```python
from build123d import *

# Parameters (mm, degrees)
F3_R     = 1.75
F4_DEPTH = 12.5
F6_R     = 2
F8_DEPTH = 10
F2_W     = 25.478227
F2_H     = 5.5
F9_DEPTH = 1.3
F10_R    = 1


with BuildPart() as f1:
    # F0 (on Front) → F1 (revolve)
    with BuildSketch(Plane.XZ):
        Polygon((-9, -6), (0, -6), (0, 3), (-5, 3), (-5, -2), (-9, -2), align=None)
    revolve(axis=Axis((0, 0, -1.5), (0, 0, 1)))


with BuildPart() as f4:
    # F3 (on Top) → F4 (new body, symmetric)
    with BuildSketch(Plane.XY):
        Circle(F3_R)
    extrude(amount=F4_DEPTH, both=True)


with BuildPart() as f1_1:
    add(f1.part)

    # F5: cut F4
    add(f4.part, mode=Mode.SUBTRACT)

    # F6
    f6_edges = [f1_1.edges().sort_by_distance(p)[0] for p in [
        (5, 0, -2),
    ]]
    fillet(f6_edges, radius=F6_R)

    # F7 (on Top) → F8 (cut)
    with BuildSketch(Plane.XY):
        with BuildLine():
            ThreePointArc((-7.782135, -0.892736), (-7.266714, 0), (-7.782135, 0.892736))
            Line((-7.782135, 0.892736), (-10.312837, 2.353838))
            Line((-10.312837, 2.353838), (-10.499112, 2.339878))
            Line((-10.499112, 2.339878), (-10.499112, -2.339878))
            Line((-10.499112, -2.339878), (-10.312837, -2.353838))
            Line((-10.312837, -2.353838), (-7.782135, -0.892736))
        make_face()
        with BuildLine():
            Line((-10.474608, 2.447236), (-10.312837, 2.353838))
            Line((-10.312837, 2.353838), (-7.398805, 2.572214))
            ThreePointArc((-7.398805, 2.572214), (-6.547083, 3.152909), (-6.624118, 4.180869))
            Line((-6.624118, 4.180869), (-8.270253, 6.595307))
            Line((-8.270253, 6.595307), (-8.444138, 6.663552))
            Line((-8.444138, 6.663552), (-10.474608, 2.447236))
        make_face()
        Polygon((-10.499112, 2.396354), (-10.474608, 2.447236), (-10.499112, 2.461384), align=None)
        Polygon((-10.527328, 2.337764), (-10.499112, 2.339878), (-10.499112, 2.396354), align=None)
        with BuildLine():
            Line((-7.398805, -2.572214), (-10.312837, -2.353838))
            Line((-10.312837, -2.353838), (-10.474608, -2.447236))
            Line((-10.474608, -2.447236), (-8.444138, -6.663552))
            Line((-8.444138, -6.663552), (-8.270253, -6.595307))
            Line((-8.270253, -6.595307), (-6.624118, -4.180869))
            ThreePointArc((-6.624118, -4.180869), (-6.547083, -3.152909), (-7.398805, -2.572214))
        make_face()
        Polygon((-8.470477, 6.673889), (-8.444138, 6.663552), (-8.419634, 6.714434), align=None)
        Polygon((-10.499112, -2.396354), (-10.499112, -2.339878), (-10.527328, -2.337764), align=None)
        Polygon((-10.499112, -2.461384), (-10.474608, -2.447236), (-10.499112, -2.396354), align=None)
        with BuildLine():
            Line((-8.37548, 6.749646), (-8.270253, 6.595307))
            Line((-8.270253, 6.595307), (-5.550051, 5.527706))
            ThreePointArc((-5.550051, 5.527706), (-4.530722, 5.681345), (-4.154113, 6.64093))
            Line((-4.154113, 6.64093), (-4.589644, 9.530495))
            Line((-4.589644, 9.530495), (-4.716699, 9.667427))
            Line((-4.716699, 9.667427), (-8.37548, 6.749646))
        make_face()
        Polygon((-8.391419, 6.773024), (-8.419634, 6.714434), (-8.37548, 6.749646), align=None)
        Polygon((-8.419634, -6.714434), (-8.444138, -6.663552), (-8.470477, -6.673889), align=None)
        Polygon((-8.37548, -6.749646), (-8.419634, -6.714434), (-8.391419, -6.773024), align=None)
        with BuildLine():
            Line((-5.550051, -5.527706), (-8.270253, -6.595307))
            Line((-8.270253, -6.595307), (-8.37548, -6.749646))
            Line((-8.37548, -6.749646), (-4.716699, -9.667427))
            Line((-4.716699, -9.667427), (-4.589644, -9.530495))
            Line((-4.589644, -9.530495), (-4.154113, -6.64093))
            ThreePointArc((-4.154113, -6.64093), (-4.530722, -5.681345), (-5.550051, -5.527706))
        make_face()
        Polygon((-4.735944, 9.688168), (-4.716699, 9.667427), (-4.672544, 9.702639), align=None)
        with BuildLine():
            Line((-4.617485, 9.715206), (-4.589644, 9.530495))
            Line((-4.589644, 9.530495), (-2.602041, 7.388368))
            ThreePointArc((-2.602041, 7.388368), (-1.616996, 7.084522), (-0.861334, 7.785673))
            Line((-0.861334, 7.785673), (0, 10.578051))
            Line((0, 10.578051), (-0.055059, 10.756549))
            Line((-0.055059, 10.756549), (-4.617485, 9.715206))
        make_face()
        Polygon((-4.621702, 9.743184), (-4.672544, 9.702639), (-4.617485, 9.715206), align=None)
        Polygon((-4.672544, -9.702639), (-4.716699, -9.667427), (-4.735944, -9.688168), align=None)
        Polygon((-4.617485, -9.715206), (-4.672544, -9.702639), (-4.621702, -9.743184), align=None)
        with BuildLine():
            Line((-2.602041, -7.388368), (-4.589644, -9.530495))
            Line((-4.589644, -9.530495), (-4.617485, -9.715206))
            Line((-4.617485, -9.715206), (-0.055059, -10.756549))
            Line((-0.055059, -10.756549), (0, -10.578051))
            Line((0, -10.578051), (-0.861334, -7.785673))
            ThreePointArc((-0.861334, -7.785673), (-1.616996, -7.084522), (-2.602041, -7.388368))
        make_face()
        Polygon((-0.063399, 10.783587), (-0.055059, 10.756549), (0, 10.769116), align=None)
        with BuildLine():
            Line((0.055059, 10.756549), (0, 10.578051))
            Line((0, 10.578051), (0.861334, 7.785673))
            ThreePointArc((0.861334, 7.785673), (1.616996, 7.084522), (2.602041, 7.388368))
            Line((2.602041, 7.388368), (4.589644, 9.530495))
            Line((4.589644, 9.530495), (4.617485, 9.715206))
            Line((4.617485, 9.715206), (0.055059, 10.756549))
        make_face()
        Polygon((0.063399, 10.783587), (0, 10.769116), (0.055059, 10.756549), align=None)
        Polygon((0, -10.769116), (-0.055059, -10.756549), (-0.063399, -10.783587), align=None)
        Polygon((0.055059, -10.756549), (0, -10.769116), (0.063399, -10.783587), align=None)
        with BuildLine():
            Line((0.861334, -7.785673), (0, -10.578051))
            Line((0, -10.578051), (0.055059, -10.756549))
            Line((0.055059, -10.756549), (4.617485, -9.715206))
            Line((4.617485, -9.715206), (4.589644, -9.530495))
            Line((4.589644, -9.530495), (2.602041, -7.388368))
            ThreePointArc((2.602041, -7.388368), (1.616996, -7.084522), (0.861334, -7.785673))
        make_face()
        Polygon((4.621702, 9.743184), (4.617485, 9.715206), (4.672544, 9.702639), align=None)
        with BuildLine():
            Line((4.716699, 9.667427), (4.589644, 9.530495))
            Line((4.589644, 9.530495), (4.154113, 6.64093))
            ThreePointArc((4.154113, 6.64093), (4.530722, 5.681345), (5.550051, 5.527706))
            Line((5.550051, 5.527706), (8.270253, 6.595307))
            Line((8.270253, 6.595307), (8.37548, 6.749646))
            Line((8.37548, 6.749646), (4.716699, 9.667427))
        make_face()
        Polygon((4.735944, 9.688168), (4.672544, 9.702639), (4.716699, 9.667427), align=None)
        Polygon((4.672544, -9.702639), (4.617485, -9.715206), (4.621702, -9.743184), align=None)
        Polygon((4.716699, -9.667427), (4.672544, -9.702639), (4.735944, -9.688168), align=None)
        with BuildLine():
            Line((4.154113, -6.64093), (4.589644, -9.530495))
            Line((4.589644, -9.530495), (4.716699, -9.667427))
            Line((4.716699, -9.667427), (8.37548, -6.749646))
            Line((8.37548, -6.749646), (8.270253, -6.595307))
            Line((8.270253, -6.595307), (5.550051, -5.527706))
            ThreePointArc((5.550051, -5.527706), (4.530722, -5.681345), (4.154113, -6.64093))
        make_face()
        Polygon((8.391419, 6.773024), (8.37548, 6.749646), (8.419634, 6.714434), align=None)
        with BuildLine():
            Line((8.444138, 6.663552), (8.270253, 6.595307))
            Line((8.270253, 6.595307), (6.624118, 4.180869))
            ThreePointArc((6.624118, 4.180869), (6.547083, 3.152909), (7.398805, 2.572214))
            Line((7.398805, 2.572214), (10.312837, 2.353838))
            Line((10.312837, 2.353838), (10.474608, 2.447236))
            Line((10.474608, 2.447236), (8.444138, 6.663552))
        make_face()
        Polygon((8.470477, 6.673889), (8.419634, 6.714434), (8.444138, 6.663552), align=None)
        Polygon((8.419634, -6.714434), (8.37548, -6.749646), (8.391419, -6.773024), align=None)
        Polygon((8.444138, -6.663552), (8.419634, -6.714434), (8.470477, -6.673889), align=None)
        with BuildLine():
            Line((6.624118, -4.180869), (8.270253, -6.595307))
            Line((8.270253, -6.595307), (8.444138, -6.663552))
            Line((8.444138, -6.663552), (10.474608, -2.447236))
            Line((10.474608, -2.447236), (10.312837, -2.353838))
            Line((10.312837, -2.353838), (7.398805, -2.572214))
            ThreePointArc((7.398805, -2.572214), (6.547083, -3.152909), (6.624118, -4.180869))
        make_face()
        Polygon((10.499112, 2.461384), (10.474608, 2.447236), (10.499112, 2.396354), align=None)
        with BuildLine():
            Line((10.499112, 2.339878), (10.312837, 2.353838))
            Line((10.312837, 2.353838), (7.782135, 0.892736))
            ThreePointArc((7.782135, 0.892736), (7.266714, 0), (7.782135, -0.892736))
            Line((7.782135, -0.892736), (10.312837, -2.353838))
            Line((10.312837, -2.353838), (10.499112, -2.339878))
            Line((10.499112, -2.339878), (10.499112, 2.339878))
        make_face()
        Polygon((10.527328, 2.337764), (10.499112, 2.396354), (10.499112, 2.339878), align=None)
        Polygon((10.499112, -2.396354), (10.474608, -2.447236), (10.499112, -2.461384), align=None)
        Polygon((10.499112, -2.339878), (10.499112, -2.396354), (10.527328, -2.337764), align=None)
    extrude(amount=-F8_DEPTH, mode=Mode.SUBTRACT)

    # F2 (on Top) → F9 (cut, symmetric)
    with BuildSketch(Plane.XY):
        with Locations((1.864194, 0)):
            Rectangle(F2_W, F2_H)
    extrude(amount=F9_DEPTH, both=True, mode=Mode.SUBTRACT)

    # F10
    f10_edges = [f1_1.edges().sort_by_distance(p)[0] for p in [
        (5, 0, 3),
    ]]
    fillet(f10_edges, radius=F10_R)


solid = f1_1.part
```
Geometry check sheet. Reference: the model listing, model coordinates, mm. A direction names the side the tool comes from. Coordinates: 2 decimals unless noted, no trailing zeros. Order: outer loops, then holes, each group sorted by start corner. A loop starts at its lowest first (then second) coordinate and runs counter-clockwise, first axis right, second up.
Item 1: Section check D-D (z = -0.5). Enter the section's corners in (x, y).
Item 2: Section check C-C (z = 0.5). Enter the section's corners in (x, y).
Item 3: Depth check by flat-ended pin: pin 1 (2 mm diameter, centred on x = -1, z = -0.5, fed in from +Y); pin 2 (2 mm diameter, centred on x = -1, z = 0, fed in from -Y); pin 3 (5 mm diameter, centred on x = 3, z = 2, fed in from +Y). Enter the tip coordinate at first touch or a pass-through.
Item 4: Section check B-B (y = 0). Enter the section's corners in (x, z), plus the area to 3 significant figures.
Item 5: Scan lines: line 1 along Y through (x, z) = (0, 1.85); line 2 along Z through (x, y) = (2, 0.75); line 3 along Z through (x, y) = (-4.75, 2). Record each from-to range of solid material in increasing order.
Item 6: Mould release check, pull along Y, two halves, no side actions. Record for faces 1 (the flat face through (0, 2.75, 0)), 2 (the flat face through (-3.04, 7.86, -3.97)), 3 (the flat face through (-3, 7, -2)), 4 (the cylindrical face through (4.543, -5.672, -3.972)): released by +Y, released by -Y, zero draft, split by the parting line, or undercut.
Item 7: Section check A-A (x = 0). Enter the section's corners in (y, z).
Item 8: Tool access check on faces 5 (the flat face through (6.127, 5.754, -3.972)), 6 (the cylindrical face through (3.911, 8.106, -4.028)), 7 (the flat face through (-4.25, -7.27, -3.97)), 8 (the flat face through (6.97, -4.69, -3.97)), 9 (the flat face through (0.68, -8.38, -3.97)). Record the directions out of +Z, -Z, +X, -X, +Y, -Y that give a thin tool (end or side, any length) a straight path to the whole face; none if there is none.
Check sheet entries:
1. outline: (-4.25, -2.75) arc R5.06 ccw to (4.25, -2.75) - close; (-4.25, 2.75) - (4.25, 2.75) arc R5.06 ccw to start
2. outline: (-4.18, -2.75) arc R5 ccw to (4.18, -2.75) - close; (-4.18, 2.75) - (4.18, 2.75) arc R5 ccw to start
3. pin 1: stops at y = 5.6
3. pin 2: stops at y = -5.2
3. pin 3: stops at y = 4.97
4. outline: (-7.27, -6) - (-1.75, -6) - (-1.75, -1.3) - (-5.48, -1.3) arc R2 cw to (-7, -2) - (-7.27, -2) - close; (-5, 1.3) - (-1.75, 1.3) - (-1.75, 3) - (-4, 3) arc R1 ccw to (-5, 2) - close; (1.75, -6) - (7.27, -6) - (7.27, -2) - (7, -2) arc R2 cw to (5.48, -1.3) - (1.75, -1.3) - close; (1.75, 1.3) - (5, 1.3) - (5, 2) arc R1 ccw to (4, 3) - (1.75, 3) - close
4. area: 60.6 mm2
5. line 1: y = -5 to -1.75, 1.75 to 5
5. line 2: z = -6 to -1.3, 1.3 to 3
5. line 3: z = -6 to -1.3
6. face 1: undercut
6. face 2: released by +Y
6. face 3: zero draft
6. face 4: undercut
7. outline: (-9, -6) - (-1.75, -6) - (-1.75, -1.3) - (-2.75, -1.3) - (-2.75, 1.3) - (-1.75, 1.3) - (-1.75, 3) - (-4, 3) arc R1 ccw to (-5, 2) - (-5, 0) arc R2 cw to (-7, -2) - (-9, -2) - close; (1.75, -6) - (9, -6) - (9, -2) - (7, -2) arc R2 cw to (5, 0) - (5, 2) arc R1 ccw to (4, 3) - (1.75, 3) - (1.75, 1.3) - (2.75, 1.3) - (2.75, -1.3) - (1.75, -1.3) - close
8. face 5: +Z, -Z, +Y
8. face 6: +Z, -Z, +X, +Y
8. face 7: +Z, -Z, -X
8. face 8: +Z, -Z, +X
8. face 9: +Z, -Z, -Y
